from build123d import *

# Parameters (mm, degrees)
EXTRUDE1_DEPTH     = 56
SKETCH2_R          = 1.5
CUT_EXTRUDE1_DEPTH = 26.22
SKETCH3_R          = 11
CUT_EXTRUDE2_DEPTH = 26.22
SKETCH4_R          = 1.5
CUT_EXTRUDE3_DEPTH = 26.22
SKETCH5_R          = 1.5
CUT_EXTRUDE4_DEPTH = 26.22


with BuildPart() as part:
    # Sketch1 → Extrude1 (new body)
    with BuildSketch(Plane.XY):
        Polygon((0, 0), (0, -25.22), (25.22, -25.22), (25.22, -23.8), (1.42, -23.8), (1.42, 0), align=None)
    extrude(amount=EXTRUDE1_DEPTH)

    # Sketch2 → Cut-Extrude1 (cut, through all)
    with BuildSketch(Plane.ZY):
        with Locations((21.4, -12.61)):
            Circle(SKETCH2_R)
    extrude(amount=-CUT_EXTRUDE1_DEPTH, mode=Mode.SUBTRACT)

    # Sketch3 → Cut-Extrude2 (cut, through all)
    with BuildSketch(Plane.XZ.offset(25.22)):
        with Locations((25.22, 21.4)):
            Circle(SKETCH3_R)
    extrude(amount=-CUT_EXTRUDE2_DEPTH, mode=Mode.SUBTRACT)

    # Sketch4 → Cut-Extrude3 (cut, through all)
    with BuildSketch(Plane.XZ.offset(25.22)):
        with Locations((9.72, 36.9)):
            Circle(SKETCH4_R)
    extrude(amount=-CUT_EXTRUDE3_DEPTH, mode=Mode.SUBTRACT)

    # Sketch5 → Cut-Extrude4 (cut, through all)
    with BuildSketch(Plane.XZ.offset(25.22)):
        with Locations((9.72, 5.9)):
            Circle(SKETCH5_R)
    extrude(amount=-CUT_EXTRUDE4_DEPTH, mode=Mode.SUBTRACT)


solid = part.part
Work out the finished part from the listing and answer in its coordinate system (mm). A direction names the side the tool comes from. Round coordinates to 2 decimals unless told otherwise and drop trailing zeros. Loops run counter-clockwise (first coordinate to the right, second up) from the corner with the lowest first, then second, coordinate; pieces in that order, holes last. Notation, with made-up numbers: (28, 70) - (87, 70) arc R30 cw to (87, 96) - close; hole circle Ø10 at (32.5, -39). An arc over 180 degrees is marked (long way). Use one line per item in the form item = value. Start each with the question number.
(1) Which of the six approach directions +Z, -Z, +X, -X, +Y, -Y give full straight-line access (tool end or side, diameter ignored) to faces 4 (the face through (13, -23.8, 28)), 5 (the face through (10.41, -24.52, 35.57))?
(2) Flat-ended cylindrical pins translate along their axes: P1, Ø12, axis at x = 8, z = 19.5, coming from the +Y side; P2, Ø10, axis at y = -7, z = 36.5, coming from the +X side. Find the tip coordinate at first contact, or state that the pin passes through.
(3) Find section C-C on z = 36.9. Determine the outline of the cut face in (x, y), and give its area (3 significant figures).
(4) Find section B-B on x = 9.72. Determine the outline of the cut face in (y, z), and give its area (3 significant figures).
(5) Find section A-A on y = -12.61. Determine the outline of the cut face in (x, z), and give its area (3 significant figures).
(6) Consider line 1 (Z direction, x = 9.72, y = -24.25); line 2 (Y direction, x = 0.95, z = 21.4); line 3 (X direction, y = -11.5, z = 24). Determine where each line is inside the solid, lowest interval first.
(7) Find section D-D on z = 21.4. Determine the outline of the cut face in (x, y), and give its area (3 significant figures).
(8) Determine the mould class of faces 1 (the face through (1, -16, 56)), 2 (the face through (25.22, -25, 5)), 3 (the face through (10.526, -24.52, 7.165)) for opening direction Z: +Z half, -Z half, draft (parallel to the pull), parting line (faces both ways), or undercut.
Answer list:
q1.face_4 = +Z, -Z, +X, +Y
q1.face_5 = +Y, -Y
q2.P1 = -23.8
q2.P2 = 1.42
q3.outline = (0, -25.22) - (8.22, -25.22) - (8.22, -23.8) - (1.42, -23.8) - (1.42, 0) - (0, 0) - close; (11.22, -25.22) - (25.22, -25.22) - (25.22, -23.8) - (11.22, -23.8) - close
q3.area = 65.3 mm^2
q4.outline = (-25.22, 0) - (-23.8, 0) - (-23.8, 4.4) - (-25.22, 4.4) - close; (-25.22, 7.4) - (-23.8, 7.4) - (-23.8, 35.4) - (-25.22, 35.4) - close; (-25.22, 38.4) - (-23.8, 38.4) - (-23.8, 56) - (-25.22, 56) - close
q4.area = 71.0 mm^2
q5.outline = (0, 0) - (1.42, 0) - (1.42, 19.9) - (0, 19.9) - close; (0, 22.9) - (1.42, 22.9) - (1.42, 56) - (0, 56) - close
q5.area = 75.3 mm^2
q6.line_1 = 0 to 4.4, 7.4 to 35.4, 38.4 to 56
q6.line_2 = -25.22 to -14.11, -11.11 to 0
q6.line_3 = 0 to 1.42
q7.outline = (0, -25.22) - (14.22, -25.22) - (14.22, -23.8) - (1.42, -23.8) - (1.42, -14.11) - (0, -14.11) - close; (0, -11.11) - (1.42, -11.11) - (1.42, 0) - (0, 0) - close
q7.area = 49.7 mm^2
q8.face_1 = +Z half
q8.face_2 = draft
q8.face_3 = undercut
